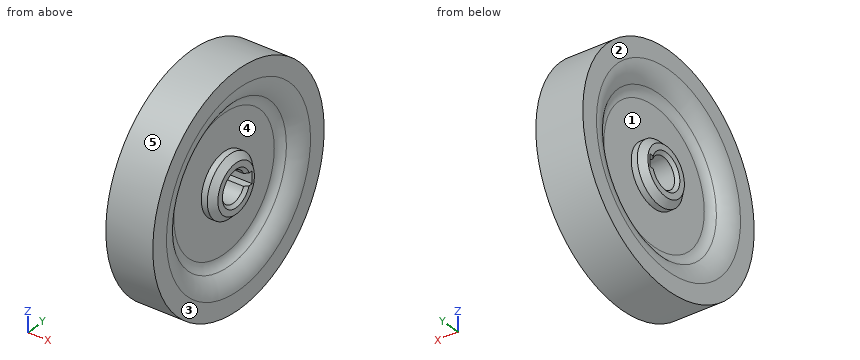
from build123d import *

# Parameters (mm, degrees)
SFAZOWANIE1_SIZE           = 2
SFAZOWANIE2_SIZE           = 2
OTW_R_10_0_10_1_D          = 10
SFAZOWANIE3_SIZE           = 1
SZKIC4_W                   = 4
SZKIC4_H                   = 4
WYTNIJ_WYCI_GNI_CIE1_DEPTH = 15.777533215


with BuildPart() as part:
    # Szkic1 → Obrót1 (revolve)
    with BuildSketch(Plane.XY, mode=Mode.PRIVATE) as obr_t1_sk:
        with BuildLine():
            Line((-7.777533215, 37.555066431), (-7.777533215, 31.555066431))
            ThreePointArc((-7.777533215, 31.555066431), (-6.938880447, 28.002476296), (-4.6, 25.2))
            ThreePointArc((-4.6, 25.2), (-3.422291236, 23.788854382), (-3, 22))
            Line((-3, 22), (-3, 10))
            Line((-3, 10), (-7, 10))
            Line((-7, 10), (-7, 0))
            Line((-7, 0), (7, 0))
            Line((7, 0), (7, 10))
            Line((7, 10), (3, 10))
            Line((3, 10), (3, 22))
            ThreePointArc((3, 22), (3.422291236, 23.788854382), (4.6, 25.2))
            ThreePointArc((4.6, 25.2), (6.938880447, 28.002476296), (7.777533215, 31.555066431))
            Line((7.777533215, 31.555066431), (7.777533215, 37.555066431))
            Line((7.777533215, 37.555066431), (-7.777533215, 37.555066431))
        make_face()
    revolve(obr_t1_sk.sketch.rotate(Axis((-1.77338341, 0, 0), (1, 0, 0)), 90), axis=Axis((-1.77338341, 0, 0), (1, 0, 0)))  # turned: the seam where the file's is

    # Sfazowanie1
    sfazowanie1_edges = [part.edges().sort_by_distance(p)[0] for p in [
        (7, 0, -10),
    ]]
    chamfer(sfazowanie1_edges, length=SFAZOWANIE1_SIZE)

    # Sfazowanie2
    sfazowanie2_edges = [part.edges().sort_by_distance(p)[0] for p in [
        (-7, 0, -10),
    ]]
    chamfer(sfazowanie2_edges, length=SFAZOWANIE2_SIZE)

    # Otwór Ø10.0 (10)1 (through all)
    with Locations(Plane.ZY.offset(7)):
        with Locations((0, 0)):
            Hole(OTW_R_10_0_10_1_D / 2)

    # Sfazowanie3
    sfazowanie3_edges = [part.edges().sort_by_distance(p)[0] for p in [
        (7, 0, 5),
        (-7, 0, 5),
    ]]
    chamfer(sfazowanie3_edges, length=SFAZOWANIE3_SIZE)

    # Szkic4 → Wytnij-wyciągnięcie1 (cut, through all)
    with BuildSketch(Plane(origin=(7, 0, 0), x_dir=(0, 0, -1), z_dir=(1, 0, 0))):
        with Locations((0, 5)):
            Rectangle(SZKIC4_W, SZKIC4_H)
    extrude(amount=-WYTNIJ_WYCI_GNI_CIE1_DEPTH, mode=Mode.SUBTRACT)


solid = part.part
Model file for the job. Use its own axes, mm. Face numbers are marked on the shaded views. A direction names the side the tool comes from. Give positions to 0.01 mm unless a question says otherwise; leave off trailing zeros. Order: outer loops, then holes, each group sorted by start corner. A loop starts at its lowest first (then second) coordinate and runs counter-clockwise, first axis right, second up. Notation, with made-up numbers: (-0.75, -37) -> (54.25, -37) arc R23 cw to (54.25, -5) -> close; hole circle Ø9 at (18, -6.5). An arc over 180 degrees is marked (long way). Use CSV: the item, a comma, the result in double quotes.
1. Mould opens along Z. For the marked faces 3, 4 and 5 say: +Z half, -Z half, draft (parallel to the pull), parting line (faces both ways), or undercut.
Outcome:
face 3,"draft"
face 4,"undercut"
face 5,"parting line"
2. 3-axis set-ups, long thin cutter, end or side, ignore diameter. For the marked faces 1 and 2: which of +Z, -Z, +X, -X, +Y, -Y reach the whole face in a straight line?
Outcome:
face 1,"-X"
face 2,"+Z, -Z, -X, +Y, -Y"
3. Band-saw the part on B-B, the plane x = -2. Give the cut face in (y, z).
Outcome:
outline,"circle Ø75.11 at (0, 0); hole (4.58, -2) -> (7, -2) -> (7, 2) -> (4.58, 2) arc R5 ccw (long way) to start"
4. Band-saw the part on C-C, the plane z = 32.5. Give the cut face in (x, y).
Outcome:
outline,"(-7.78, -18.82) -> (7.78, -18.82) -> (7.78, 18.82) -> (-7.78, 18.82) -> close"
5. Drop flat-ended pins along their axis: pin 1 (6 mm diameter, centred on x = 4, y = -17, fed in from +Z); pin 2 (1.2 mm diameter, centred on x = -1.5, y = 5.5, fed in from -Z); pin 3 (2 mm diameter, centred on x = -1, y = -19, fed in from +Z); pin 4 (9 mm diameter, centred on y = 0, z = 0, fed in from -X). Give the stop position or say it passes through.
Outcome:
pin 1,"z = 34.85"
pin 2,"z = -37.23"
pin 3,"z = 32.96"
pin 4,"through"
6. Drill centre lines: line 1 along Y through (x, z) = (-0.25, 0); line 2 along Z through (x, y) = (-6.75, 2.5); line 3 along X through (y, z) = (17, 6.5). Where is each one in solid material? Low to high. Write a range as from..to.
Outcome:
line 1,"-37.56..-5, 7..37.56"
line 2,"-37.47..-27.53, -7.86..-5.18, 5.18..7.86, 27.53..37.47"
line 3,"-3..3"
